Study the drawing (mm; zero at the part's minimum x, y, z) and answer. A direction names the side the tool comes from. Coordinates: 2 decimals unless noted, no trailing zeros. Write each loop counter-clockwise with the first axis right and the second up, starting at its lowest first coordinate (ties: lowest second). Pieces come first, ordered by that corner, then holes. Notation, with made-up numbers: (-33, 12.5) - (-10, 12.5) arc R17 cw to (-10, 23.5) - close; hole circle Ø11 at (63, 66). An arc over 180 degrees is marked (long way). One line per item, written item: value.
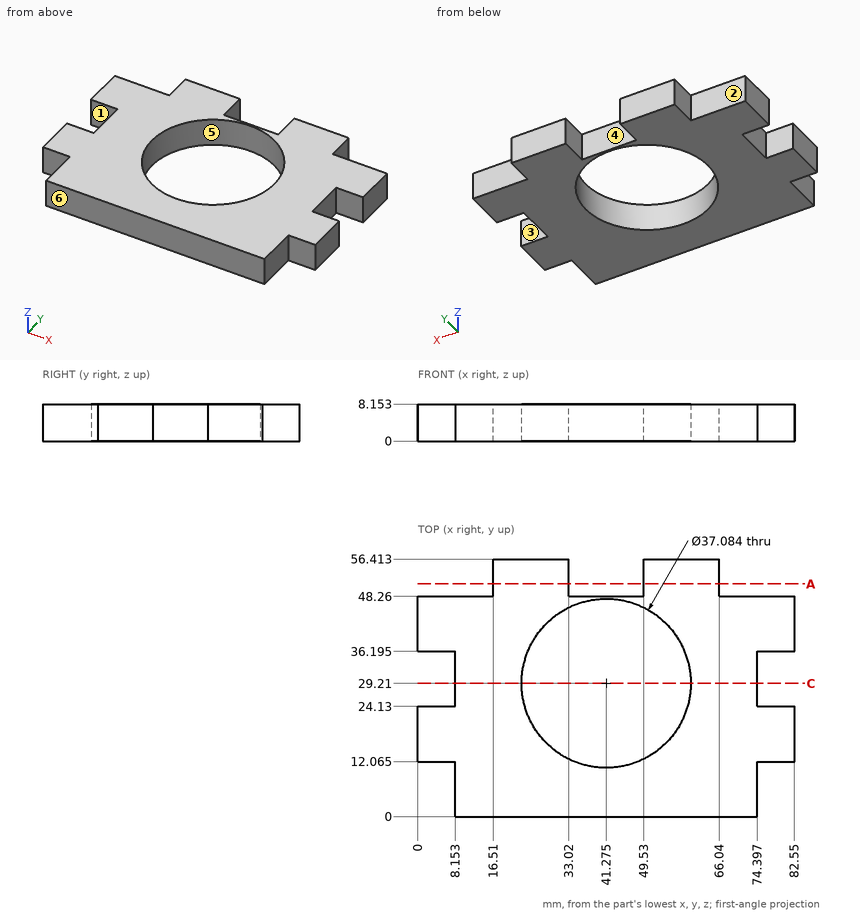
Item 1: Section C-C, the plane y = 29.21 is taken. Determine the outline of the cut face in (x, z).
Evaluation:
outline: (8.15, 0) - (22.73, 0) - (22.73, 8.15) - (8.15, 8.15) - close; (59.82, 0) - (74.4, 0) - (74.4, 8.15) - (59.82, 8.15) - close
Item 2: Section A-A, the plane y = 51 is taken. Determine the outline of the cut face in (x, z).
Evaluation:
outline: (16.51, 0) - (33.02, 0) - (33.02, 8.15) - (16.51, 8.15) - close; (49.53, 0) - (66.04, 0) - (66.04, 8.15) - (49.53, 8.15) - close
Item 3: Consider probe 1 along X at (y, z) = (51, 4); probe 2 along Y at (x, z) = (79, 5) (1 decimal); probe 3 along X at (y, z) = (29, 2.5) (1 decimal). Determine where each line is inside the solid, lowest interval first.
Evaluation:
probe 1: x = 16.51 to 33.02, 49.53 to 66.04
probe 2: y = 12.1 to 24.1, 36.2 to 48.3
probe 3: x = 8.2 to 22.7, 59.8 to 74.4
Item 4: Determine the mould class of the marked faces 4, 5 and 6 for opening direction Y: +Y half, -Y half, draft (parallel to the pull), parting line (faces both ways), or undercut.
Evaluation:
face 4: +Y half
face 5: undercut
face 6: -Y half
Item 5: Given pin 1 (4 mm diameter, centred on x = 6, z = 4.5, fed in from +Y); pin 2 (4 mm diameter, centred on x = 77.5, z = 4.5, fed in from -Y) (1 decimal); pin 3 (2.5 mm diameter, centred on y = 29, z = 5, fed in from -X), each flat-ended and moving along its own axis, determine where each tip first touches the part or whether it passes through.
Evaluation:
pin 1: stops at y = 48.26
pin 2: stops at y = 12.1
pin 3: stops at x = 8.15
Item 6: Which of the six approach directions +Z, -Z, +X, -X, +Y, -Y give full straight-line access (tool end or side, diameter ignored) to the marked faces 1, 2 and 3?
Evaluation:
face 1: +Z, -Z, -X
face 2: +Z, -Z, -X, +Y
face 3: +Z, -Z, +X
